from build123d import *

# Parameters (mm, degrees)
SKETCH1_R           = 4.775
BOSS_EXTRUDE1_DEPTH = 50
CUT_EXTRUDE2_DEPTH  = 8
CHAMFER2_SIZE       = 0.75


with BuildPart() as part:
    # Sketch1 → Boss-Extrude1 (new body)
    with BuildSketch(Plane(origin=(0, 0, 0), x_dir=(1, 0, 0), z_dir=(0, 1, 0))):
        with Locations(Location((0, 0, 0), (0, 0, 270))):
            Circle(SKETCH1_R)
    extrude(amount=BOSS_EXTRUDE1_DEPTH)

    # Sketch3 → Cut-Extrude2 (cut)
    with BuildSketch(Plane.XZ):
        with BuildLine():
            ThreePointArc((5.7947785, 0), (4.752316007, 3.315863452), (2, 5.438700016))
            Line((2, 5.438700016), (2, 4.33596875))
            ThreePointArc((2, 4.33596875), (4.021854361, 2.57396824), (4.775, 0))
            ThreePointArc((4.775, 0), (4.021854361, -2.57396824), (2, -4.33596875))
            Line((2, -4.33596875), (2, -5.438700016))
            ThreePointArc((2, -5.438700016), (4.752316007, -3.315863452), (5.7947785, 0))
        make_face()
        with BuildLine():
            ThreePointArc((4.775, 0), (4.021854361, 2.57396824), (2, 4.33596875))
            Line((2, 4.33596875), (2, -4.33596875))
            ThreePointArc((2, -4.33596875), (4.021854361, -2.57396824), (4.775, 0))
        make_face()
        with BuildLine():
            Line((-2, -4.33596875), (-2, 4.33596875))
            ThreePointArc((-2, 4.33596875), (-4.775, 0), (-2, -4.33596875))
        make_face()
        with BuildLine():
            Line((-2, 4.33596875), (-2, 5.438700016))
            ThreePointArc((-2, 5.438700016), (-5.7947785, 0), (-2, -5.438700016))
            Line((-2, -5.438700016), (-2, -4.33596875))
            ThreePointArc((-2, -4.33596875), (-4.775, 0), (-2, 4.33596875))
        make_face()
    extrude(amount=-CUT_EXTRUDE2_DEPTH, mode=Mode.SUBTRACT)

    # Chamfer2
    chamfer2_edges = [part.edges().sort_by_distance(p)[0] for p in [
        (-2, 0, 0),
        (2, 0, 0),
    ]]
    chamfer(chamfer2_edges, length=CHAMFER2_SIZE)


solid = part.part
The listing builds one solid part. Answer for the finished solid, in the listing's coordinates (mm). A direction names the side the tool comes from. Give positions to 0.01 mm unless a question says otherwise; leave off trailing zeros. Write each loop counter-clockwise with the first axis right and the second up, starting at its lowest first coordinate (ties: lowest second). Pieces come first, ordered by that corner, then holes.
Item 1: Section C-C, the plane x = 4.25 is taken. Write down the section's boundary in (y, z), plus the area to 3 significant figures.
Item 2: Section B-B, the plane y = 32 is taken. Write down the section's boundary in (x, z) (3 decimals).
Item 3: Section A-A, the plane z = 0 is taken. Write down the section's boundary in (x, y) (3 decimals).
Item 4: Find the intervals of material crossed by line 1 along Y through (x, z) = (-3.5, 2); line 2 along Z through (x, y) = (-2, 36), in increasing order.
Item 5: Flat-ended cylindrical pins translate along their axes: P1, Ø2, axis at y = 4, z = -0.5, coming from the +X side; P2, Ø3.5, axis at y = 6, z = -0.5, coming from the -X side; P3, Ø1.5, axis at x = 1, y = 15.5, coming from the -Z side. Find the tip coordinate at first contact, or state that the pin passes through.
Item 6: Which of the six approach directions +Z, -Z, +X, -X, +Y, -Y give full straight-line access (tool end or side, diameter ignored) to faces 1 (the flat face through (0, 50, 0)), 2 (the flat face through (-2, 4, 0)), 3 (the flat face through (2, 4, 0))?
Completed:
1. outline: (8, -2.18) - (50, -2.18) - (50, 2.18) - (8, 2.18) - close
1. area: 183 mm2
2. outline: circle Ø9.55 at (0, 0)
3. outline: (-4.775, 8) - (-2, 8) - (-2, 0.75) - (-1.25, 0) - (1.25, 0) - (2, 0.75) - (2, 8) - (4.775, 8) - (4.775, 50) - (-4.775, 50) - close
4. line 1: y = 8 to 50
4. line 2: z = -4.34 to 4.34
5. P1: stops at x = 2
5. P2: stops at x = -2
5. P3: stops at z = -4.77
6. face 1: +Z, -Z, +X, -X, +Y
6. face 2: +Z, -Z, -X, -Y
6. face 3: +Z, -Z, +X, -Y
